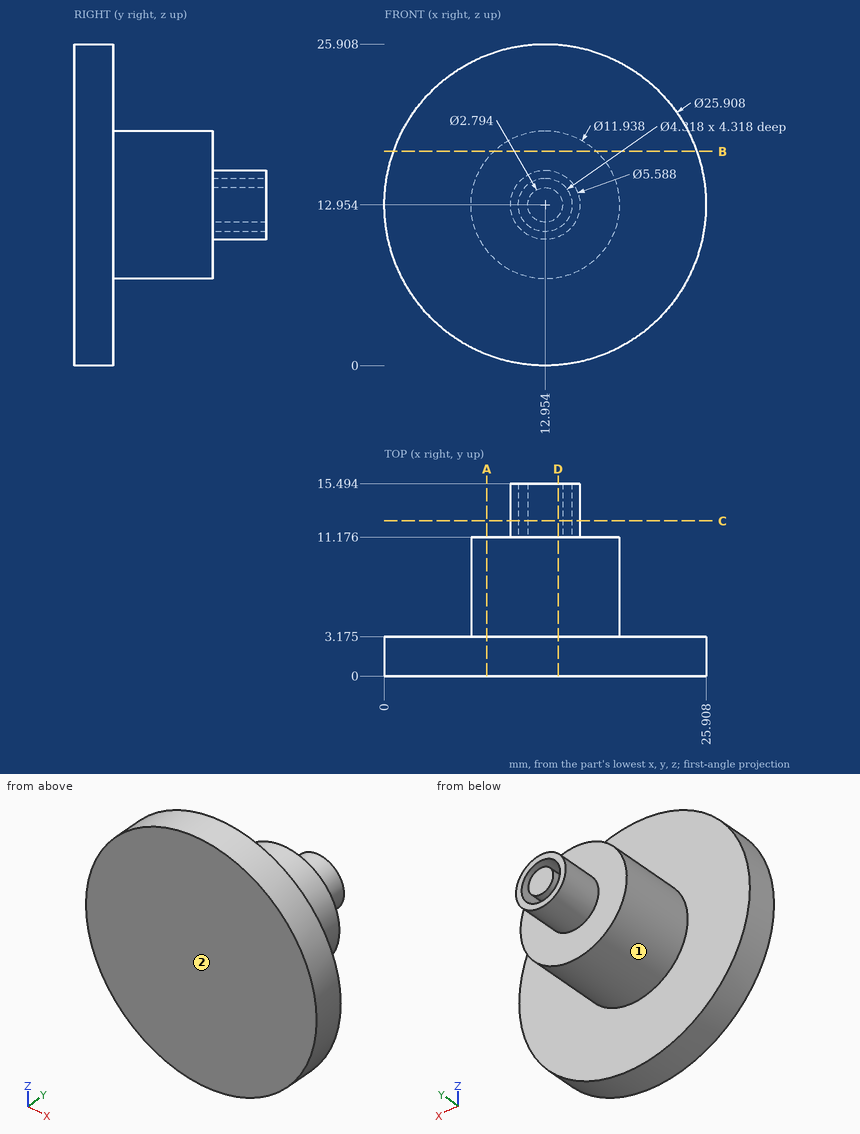
Geometry check sheet. Reference: drawing and pictorial views, mm from the part's lowest x, y, z. A direction names the side the tool comes from. Coordinates: 2 decimals unless noted, no trailing zeros. Write each loop counter-clockwise with the first axis right and the second up, starting at its lowest first coordinate (ties: lowest second). Pieces come first, ordered by that corner, then holes. Notation, with made-up numbers: (-18, -20) -> (28, -20) arc R30 cw to (28, 17) -> close; hole circle Ø8 at (-39.75, 68). An arc over 180 degrees is marked (long way). Use a Markdown table: item, result.
1. Sectioned sample at A-A (x = 8.25). Enter the section's corners in (y, z) (3 decimals).
Reported:
| item | result |
|---|---|
| outline | (0, 0.884) -> (3.175, 0.884) -> (3.175, 9.28) -> (11.176, 9.28) -> (11.176, 16.628) -> (3.175, 16.628) -> (3.175, 25.024) -> (0, 25.024) -> close |
2. Sectioned sample at D-D (x = 14). Enter the section's corners in (y, z) (3 decimals), plus the area to 3 significant figures.
Reported:
| item | result |
|---|---|
| outline | (0, 0.042) -> (3.175, 0.042) -> (3.175, 7.077) -> (11.176, 7.077) -> (11.176, 10.363) -> (15.494, 10.363) -> (15.494, 11.065) -> (11.176, 11.065) -> (11.176, 12.028) -> (15.494, 12.028) -> (15.494, 13.88) -> (11.176, 13.88) -> (11.176, 14.843) -> (15.494, 14.843) -> (15.494, 15.545) -> (11.176, 15.545) -> (11.176, 18.831) -> (3.175, 18.831) -> (3.175, 25.866) -> (0, 25.866) -> close |
| area | 190 mm2 |
3. Sectioned sample at C-C (y = 12.5). Enter the section's corners in (x, z).
Reported:
| item | result |
|---|---|
| outline | circle Ø5.59 at (12.95, 12.95); circle Ø2.79 at (12.95, 12.95); hole circle Ø4.32 at (12.95, 12.95) |
4. Sectioned sample at B-B (z = 17.25). Enter the section's corners in (x, y) (3 decimals), plus the area to 3 significant figures.
Reported:
| item | result |
|---|---|
| outline | (0.733, 0) -> (25.175, 0) -> (25.175, 3.175) -> (17.098, 3.175) -> (17.098, 11.176) -> (8.81, 11.176) -> (8.81, 3.175) -> (0.733, 3.175) -> close |
| area | 144 mm2 |
5. Tool access check on the marked faces 1 and 2. Record the directions out of +Z, -Z, +X, -X, +Y, -Y that give a thin tool (end or side, any length) a straight path to the whole face; none if there is none.
Reported:
| item | result |
|---|---|
| face 1 | +Y |
| face 2 | +Z, -Z, +X, -X, -Y |
6. Scan lines: line 1 along X through (y, z) = (11.5, 13.25); line 2 along Y through (x, z) = (11.75, 6.25) (3 decimals); line 3 along Y through (x, z) = (8.5, 11.25). Record each from-to range of solid material in increasing order.
Reported:
| item | result |
|---|---|
| line 1 | x = 10.18 to 10.82, 11.59 to 14.32, 15.09 to 15.73 |
| line 2 | y = 0 to 3.175 |
| line 3 | y = 0 to 11.18 |
7. Go/stop test with flat-tipped pins: pin 1 Ø4 at (x, y) = (3.5, 4) entering from +Z; pin 2 Ø3 at (y, z) = (6.5, 12.5) entering from -X (3 decimals); pin 3 Ø1 at (y, z) = (11, 18.5) entering from -X. Record where each tip stops, or that it passes through.
Reported:
| item | result |
|---|---|
| pin 1 | stops at z = 23.42 |
| pin 2 | stops at x = 6.985 |
| pin 3 | stops at x = 9.77 |
